Can you work these out from the drawing? Everything is in mm from the part's minimum corner. Give positions to 0.01 mm unless a question says otherwise; leave off trailing zeros. Write each loop counter-clockwise with the first axis right and the second up, starting at its lowest first coordinate (ties: lowest second). Pieces come first, ordered by that corner, then holes. Notation, with made-up numbers: (17.5, -5) - (21.5, -5) arc R27 ccw to (21.5, 33) - close; hole circle Ø6 at (-4.5, -16.75). An arc over 180 degrees is marked (long way). Use a Markdown table: item, result.
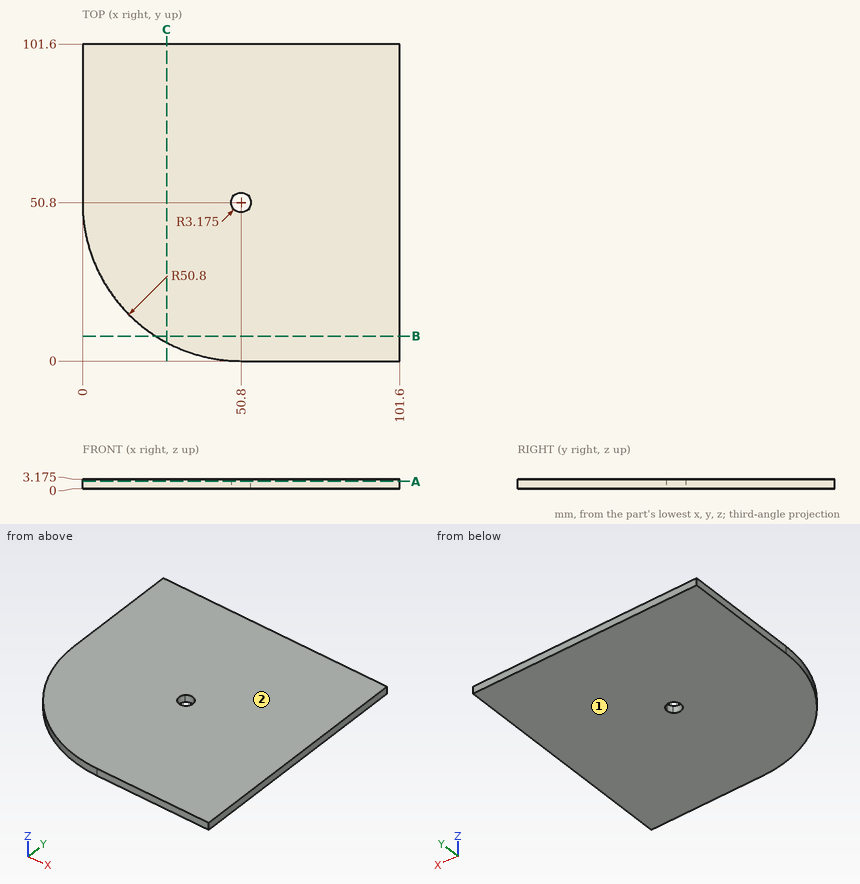
Item 1: If we section it at B-B, the plane y = 8: Write out the boundary of the cut face in (x, z) (3 decimals), plus the area to 3 significant figures.
Values:
| item | result |
|---|---|
| outline | (23.436, 0) - (101.6, 0) - (101.6, 3.175) - (23.436, 3.175) - close |
| area | 248 mm2 |
Item 2: Will this pin go through, and if not, where does the flat tip stop? pin 1 Ø1.5 at (x, z) = (15, 1.5) entering from -Y.
Values:
| item | result |
|---|---|
| pin 1 | stops at y = 14.03 |
Item 3: I need wall thicknesses on line 1 along X through (y, z) = (51, 1.2); line 2 along Y through (x, z) = (52.5, 2.85). Which ranges of each line are inside material? Lowest first, please. Write a range as [from, to].
Values:
| item | result |
|---|---|
| line 1 | x = [0, 47.63], [53.97, 101.6] |
| line 2 | y = [0, 48.12], [53.48, 101.6] |
Item 4: Thinking about a two-plate mould opening in Z: for the marked faces 1 and 2, which applies, +Z half, -Z half, draft (parallel to the pull), parting line (faces both ways), or undercut?
Values:
| item | result |
|---|---|
| face 1 | -Z half |
| face 2 | +Z half |
Item 5: If we section it at C-C, the plane x = 27: Write out the boundary of the cut face in (y, z) (3 decimals).
Values:
| item | result |
|---|---|
| outline | (5.92, 0) - (101.6, 0) - (101.6, 3.175) - (5.92, 3.175) - close |
Item 6: If we section it at A-A, the plane z = 2.45: Write out the boundary of the cut face in (x, y) (3 decimals), plus the area to 3 significant figures.
Values:
| item | result |
|---|---|
| outline | (0, 50.8) arc R50.8 ccw to (50.8, 0) - (101.6, 0) - (101.6, 101.6) - (0, 101.6) - close; hole circle Ø6.35 at (50.8, 50.8) |
| area | 9,740 mm2 |
